Check sheet for the drawn part. Datum: minimum x, y, z corner. Units: mm. A direction names the side the tool comes from. Give positions to 0.01 mm unless a question says otherwise; leave off trailing zeros. Order: outer loops, then holes, each group sorted by start corner. A loop starts at its lowest first (then second) coordinate and runs counter-clockwise, first axis right, second up. Notation, with made-up numbers: (27, 17) -> (42, 17) arc R21 ccw to (42, 50) -> close; hole circle Ø3 at (-0.5, -30.5). An arc over 180 degrees is marked (long way). Return JSON: item names as keys, results as strings. Group by question number.
(1) Cross-section at C-C on z = 22. Enter the section's corners in (x, y), then the cut area to 3 significant figures.
(2) Cross-section at A-A on y = 52. Enter the section's corners in (x, z).
(3) Cross-section at D-D on y = 43.5. Enter the section's corners in (x, z).
(4) Depth check by flat-ended pin: pin 1 Ø8 at (y, z) = (50.5, 17) entering from +X; pin 2 Ø2 at (x, y) = (11.5, 28) entering from +Z. Enter the tip coordinate at first touch or a pass-through.
(5) Thickness scan on line 1 along Z through (x, y) = (22.5, 3.5); line 2 along Y through (x, z) = (7, 34.5). Record the ranges inside material, lowest first.
(6) Cross-section at B-B on x = 51. Enter the section's corners in (y, z).
(7) Tool access check on the marked faces 1 and 2. Record the directions out of +Z, -Z, +X, -X, +Y, -Y that give a thin tool (end or side, any length) a straight path to the whole face; none if there is none.
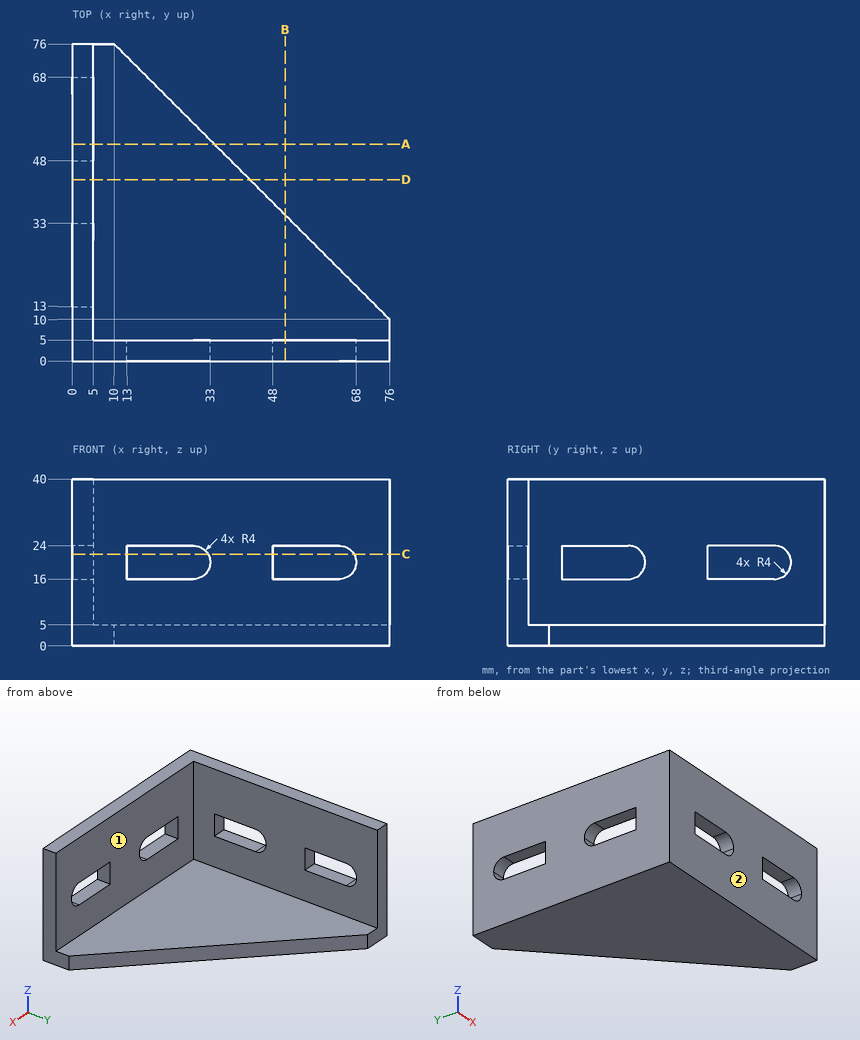
Verdict:
{
 "1": {"outline": "(0, 0) -> (13, 0) -> (13, 5) -> (5, 5) -> (5, 13) -> (0, 13) -> close; (0, 32.46) -> (5, 32.46) -> (5, 48) -> (0, 48) -> close; (0, 67.46) -> (5, 67.46) -> (5, 76) -> (0, 76) -> close; (32.46, 0) -> (48, 0) -> (48, 5) -> (32.46, 5) -> close; (67.46, 0) -> (76, 0) -> (76, 5) -> (67.46, 5) -> close", "area": "346 mm²"},
 "2": {"outline": "(0, 0) -> (34, 0) -> (34, 5) -> (5, 5) -> (5, 16) -> (0, 16) -> close; (0, 24) -> (5, 24) -> (5, 40) -> (0, 40) -> close"},
 "3": {"outline": "(0, 0) -> (42.5, 0) -> (42.5, 5) -> (5, 5) -> (5, 40) -> (0, 40) -> close"},
 "4": {"pin 1": "x = 5", "pin 2": "z = 5"},
 "5": {"line 1": "0 to 16, 24 to 40", "line 2": "0 to 5"},
 "6": {"outline": "(0, 0) -> (35, 0) -> (35, 5) -> (5, 5) -> (5, 16) -> (0, 16) -> close; (0, 24) -> (5, 24) -> (5, 40) -> (0, 40) -> close"},
 "7": {"face 1": "+Z, +X, +Y", "face 2": "+Z, -Z, +X, -X, -Y"}
}
